Geometry: final body of the model. Coordinates: model frame, mm. A direction names the side the tool comes from. Give positions to 0.01 mm unless a question says otherwise; leave off trailing zeros. Loops run counter-clockwise (first coordinate to the right, second up) from the corner with the lowest first, then second, coordinate; pieces in that order, holes last. Notation, with made-up numbers: (18, 9.25) -> (33, 9.25) arc R23 cw to (33, 48.25) -> close; hole circle Ø1 at (47.25, 28.25). An arc over 180 degrees is marked (long way). One line per question, with ' | ' between items. Start each with the question number.
Item 1: Material intervals for line 1 along Y through (x, z) = (7, 9); line 2 along Y through (x, z) = (11.5, 9.5); line 3 along X through (y, z) = (16.75, 10.25) (3 decimals), sorted ascending. Write a range as [from, to].
Item 2: Section A-A on y = 15. Return loops of the section in (x, z) (3 decimals), then the cut area to 4 significant figures.
Item 3: Mould query, pull axis Y, two halves, no side actions, for faces 4 (the flat face through (0, 6, 6)), 5 (the flat face through (7, 0, 6)), 6 (the flat face through (3, 12, 6)), 7 (the cylindrical face through (7.467, 16.054, 3.672)). Classes: released by +Y, released by -Y, zero draft, split by the parting line, or undercut.
Item 4: Section B-B on z = 9. Return loops of the section in (x, y) (3 decimals).
Item 5: Set-up query: faces 1 (the flat face through (5.125, 15, 6)), 2 (the flat face through (7, 7, 0)), 3 (the flat face through (12, 12, 6)). Return all of +Z, -Z, +X, -X, +Y, -Y with unobstructed straight access to the full face (end or side cutting, diameter ignored); none if empty.
Item 6: Section C-C on x = 7.75. Return loops of the section in (y, z).
Item 7: Section D-D on z = 6.5. Return loops of the section in (x, y) (3 decimals).
Item 8: Pin query (flat end, axial travel): P1, Ø4.5, axis at y = 15, z = 7.5, coming from the +X side (3 decimals); P2, Ø3, axis at y = 14, z = 6.5, coming from the -X side (3 decimals); P3, Ø1.5, axis at x = 3, z = 6, coming from the +Y side. Return the tip coordinate at first contact, or that it passes through.
from build123d import *

# Parameters (mm, degrees)
SKETCH1_W           = 4.75
SKETCH1_H           = 5.75
SKETCH1_W_2         = 15
SKETCH1_H_2         = 12
BOSS_EXTRUDE1_DEPTH = 12
SKETCH2_R           = 1.25
CUT_EXTRUDE1_DEPTH  = 10


with BuildPart() as part:
    # Sketch1 → Boss-Extrude1 (new body)
    with BuildSketch(Plane.XY):
        with Locations((7.5, 14.875)):
            Rectangle(SKETCH1_W, SKETCH1_H)
        with Locations((7.5, 6)):
            Rectangle(SKETCH1_W_2, SKETCH1_H_2)
    extrude(amount=BOSS_EXTRUDE1_DEPTH)

    # Sketch2 → Cut-Extrude1 (cut)
    with BuildSketch(Plane.ZY.offset(-5.125)):
        with Locations((3, 15)):
            Circle(SKETCH2_R)
        with Locations((9, 15)):
            Circle(SKETCH2_R)
    extrude(amount=-CUT_EXTRUDE1_DEPTH, mode=Mode.SUBTRACT)


solid = part.part
Result sheet:
1) line 1: y = [0, 13.75], [16.25, 17.75] | line 2: y = [0, 12] | line 3: x = [5.125, 9.875]
2) outline: (5.125, 0) -> (9.875, 0) -> (9.875, 1.75) -> (5.125, 1.75) -> close; (5.125, 4.25) -> (9.875, 4.25) -> (9.875, 7.75) -> (5.125, 7.75) -> close; (5.125, 10.25) -> (9.875, 10.25) -> (9.875, 12) -> (5.125, 12) -> close | area: 33.25 mm²
3) face 4: zero draft | face 5: released by -Y | face 6: released by +Y | face 7: undercut
4) outline: (0, 0) -> (15, 0) -> (15, 12) -> (9.875, 12) -> (9.875, 13.75) -> (5.125, 13.75) -> (5.125, 12) -> (0, 12) -> close; (5.125, 16.25) -> (9.875, 16.25) -> (9.875, 17.75) -> (5.125, 17.75) -> close
5) face 1: +Z, -Z, -X, +Y | face 2: -Z, +X, -X, +Y, -Y | face 3: +Z, -Z, +X, +Y
6) outline: (0, 0) -> (17.75, 0) -> (17.75, 12) -> (0, 12) -> close; hole circle Ø2.5 at (15, 3); hole circle Ø2.5 at (15, 9)
7) outline: (0, 0) -> (15, 0) -> (15, 12) -> (9.875, 12) -> (9.875, 17.75) -> (5.125, 17.75) -> (5.125, 12) -> (0, 12) -> close
8) P1: stops at x = 9.875 | P2: stops at x = 5.125 | P3: stops at y = 12
